Verification items for the finished model (mm, model axes). A direction names the side the tool comes from. Coordinates: 2 decimals unless noted, no trailing zeros. Order: outer loops, then holes, each group sorted by start corner. A loop starts at its lowest first (then second) coordinate and runs counter-clockwise, first axis right, second up. Notation, with made-up numbers: (45.25, 20.5) -> (88.25, 20.5) arc R16 ccw to (88.25, 43.5) -> close; hole circle Ø2 at (-4, -6.75). An arc over 180 degrees is marked (long way). Write each question's results on one line, items separated by ' | '. Start each with the question number.
(1) Thickness scan on probe 1 along Y at (x, z) = (4.95, 0); probe 2 along Y at (x, z) = (8, -1); probe 3 along X at (y, z) = (-0.5, 1.5). Record the ranges inside material, lowest first. Write a range as [from, to].
(2) Cross-section at C-C on x = 0.75. Enter the section's corners in (y, z).
(3) Draft check along Y on faces 3 (the cylindrical face through (4.73, -3.905, 0.867)), 4 (the flat face through (3, 0, 0)), 5 (the flat face through (0, 0, 0)). Enter one of: +Y half, -Y half, draft (parallel to the pull), parting line (faces both ways), or undercut.
(4) Go/stop test with a flat-tipped pin: pin 1 (1.5 mm diameter, centred on x = 8, y = -1, fed in from -Z). Record where the tip stops, or that it passes through.
(5) Set-up check for faces 1 (the flat face through (9, 2, -2)), 2 (the cylindrical face through (6.04, -2.44, 0.54)): record each of +Z, -Z, +X, -X, +Y, -Y from which the full face is reachable in a straight line by a thin tool's end or side.
(6) Cross-section at A-A on y = 0. Enter the section's corners in (x, z), and give its area (3 significant figures).
(7) Cross-section at D-D on x = 3.5. Enter the section's corners in (y, z), and give its area (3 significant figures).
```python
from build123d import *

# Parameters (mm, degrees)
SKETCH1_R           = 4
BOSS_EXTRUDE1_DEPTH = 9
CHAMFER1_SIZE       = 1
CHAMFER1_SIZE2      = 0.577350269
SKETCH2_R           = 2.5
CUT_EXTRUDE1_DEPTH  = 6


with BuildPart() as part:
    # Sketch1 → Boss-Extrude1 (new body)
    with BuildSketch(Plane(origin=(0, 0, 0), x_dir=(0, 0, -1), z_dir=(1, 0, 0))):
        Circle(SKETCH1_R)
    extrude(amount=BOSS_EXTRUDE1_DEPTH)

    # Chamfer1
    chamfer1_edges = [part.edges().sort_by_distance(p)[0] for p in [
        (0, 0, 4),
    ]]
    chamfer1_side = [part.faces().sort_by_distance(p)[0] for p in [
        (0, 0, 0),
    ]]
    chamfer(chamfer1_edges, length=CHAMFER1_SIZE, length2=CHAMFER1_SIZE2, reference=chamfer1_side[0])

    # Sketch2 → Cut-Extrude1 (cut)
    with BuildSketch(Plane(origin=(9, 0, 0), x_dir=(0, 0, -1), z_dir=(1, 0, 0))):
        Circle(SKETCH2_R)
    extrude(amount=-CUT_EXTRUDE1_DEPTH, mode=Mode.SUBTRACT)


solid = part.part
```
Results are:
1) probe 1: y = [-4, -2.5], [2.5, 4] | probe 2: y = [-3.87, -2.29], [2.29, 3.87] | probe 3: x = [0, 3]
2) outline: circle Ø8 at (0, 0)
3) face 3: parting line | face 4: undercut | face 5: draft
4) pin 1: stops at z = -3.99
5) face 1: +Z, -Z, +X, +Y, -Y | face 2: +X
6) outline: (0, -3) -> (0.58, -4) -> (9, -4) -> (9, -2.5) -> (3, -2.5) -> (3, 2.5) -> (9, 2.5) -> (9, 4) -> (0.58, 4) -> (0, 3) -> close | area: 41.4 mm2
7) outline: circle Ø8 at (0, 0); hole circle Ø5 at (0, 0) | area: 30.6 mm2
